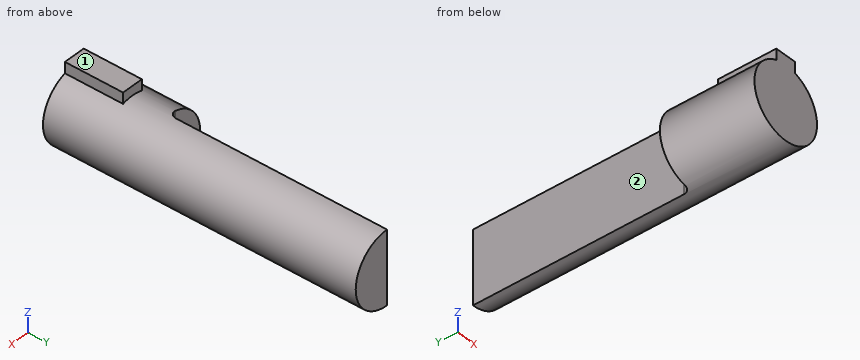
```python
from build123d import *

# Parameters (mm, degrees)
F0_R     = 5
F1_DEPTH = 43
F3_DEPTH = 8
F4_W     = 6.116576
F4_H     = 10
F5_DEPTH = 30
F6_R     = 1


with BuildPart() as f1:
    # F0 (on Front) → F1 (new body)
    with BuildSketch(Plane.XZ):
        Circle(F0_R)
    extrude(amount=F1_DEPTH)

    # F2 (on face) → F3 (join)
    with BuildSketch(Plane.XZ.offset(43)):
        with BuildLine():
            Line((-1.5, 6.269696), (-1.5, 4.769696))
            ThreePointArc((-1.5, 4.769696), (0, 5), (1.5, 4.769696))
            Line((1.5, 4.769696), (1.5, 6.269696))
            Line((1.5, 6.269696), (-1.5, 6.269696))
        make_face()
    extrude(amount=-F3_DEPTH)

    # F4 (on face) → F5 (cut)
    with BuildSketch(Plane(origin=(0, 0, 0), x_dir=(-1, 0, 0), z_dir=(0, 1, 0))):
        with Locations((3.058288, 0)):
            Rectangle(F4_W, F4_H)
    extrude(amount=-F5_DEPTH, mode=Mode.SUBTRACT)

    # F6
    f6_edges = [f1.edges().sort_by_distance(p)[0] for p in [
        (0, -30, 0),
    ]]
    fillet(f6_edges, radius=F6_R)


solid = f1.part
```
Could you check a few things on this model? Use its own coordinates, in mm. Face numbers are marked on the shaded views. A direction names the side the tool comes from. Coordinates: 2 decimals unless noted, no trailing zeros. Write each loop counter-clockwise with the first axis right and the second up, starting at its lowest first coordinate (ties: lowest second). Pieces come first, ordered by that corner, then holes. Notation, with made-up numbers: (64, 43.25) - (77, 43.25) arc R13 ccw to (77, 58.25) - close; hole circle Ø9 at (2, 29.25). An arc over 180 degrees is marked (long way). Use a Markdown table: item, result.
Q1. Please list where these lines run through material, in increasing order: L1, parallel to Z at x = 0.25, y = -22; L2, parallel to Y at x = -1.5, z = 0.5.
Geometry check:
| item | result |
|---|---|
| L1 | z = -4.99 to 4.99 |
| L2 | y = -43 to -30 |
Q2. I'm going to push flat-ended pins straight in: pin 1 Ø6 at (x, y) = (0.5, -21.5) entering from -Z; pin 2 Ø1 at (y, z) = (-37, -1.5) entering from -X; pin 3 Ø1 at (x, y) = (-3.5, -33) entering from -Z; pin 4 Ø1.2 at (y, z) = (-38, 5.5) entering from +X. Where does each tip first touch, or does it pass through?
Geometry check:
| item | result |
|---|---|
| pin 1 | stops at z = -5 |
| pin 2 | stops at x = -4.9 |
| pin 3 | stops at z = -4 |
| pin 4 | stops at x = 1.5 |
Q3. Imagine slicing it at A-A (z = 0). List the corners of the cut face in (x, y) for me.
Geometry check:
| item | result |
|---|---|
| outline | (-5, -43) - (5, -43) - (5, 0) - (0, 0) - (0, -29) arc R1 cw to (-1, -30) - (-5, -30) - close |
Q4. Which directions (+Z, -Z, +X, -X, +Y, -Y) give clear straight access to the entire face, cutting with the end or side of a thin tool? Please do the marked faces 1 and 2.
Geometry check:
| item | result |
|---|---|
| face 1 | +Z, +X, -X, +Y, -Y |
| face 2 | +Z, -Z, -X, +Y |
Q5. Imagine slicing it at C-C (z = 1.75). List the corners of the cut face in (x, y) for me, and give its area (3 significant figures).
Geometry check:
| item | result |
|---|---|
| outline | (-4.68, -43) - (4.68, -43) - (4.68, 0) - (0, 0) - (0, -29) arc R1 cw to (-1, -30) - (-4.68, -30) - close |
| area | 263 mm2 |
Q6. Imagine slicing it at B-B (y = -34.5). List the corners of the cut face in (x, z) for me, and give its area (3 significant figures).
Geometry check:
| item | result |
|---|---|
| outline | circle Ø10 at (0, 0) |
| area | 78.5 mm2 |
Q7. Imagine slicing it at D-D (x = 2.75). List the corners of the cut face in (y, z) for me, and give its area (3 significant figures).
Geometry check:
| item | result |
|---|---|
| outline | (-43, -4.18) - (0, -4.18) - (0, 4.18) - (-43, 4.18) - close |
| area | 359 mm2 |
